Read the model definition and answer for the solid it produces. Units are mm, in the model's axes. A direction names the side the tool comes from. Give positions to 0.01 mm unless a question says otherwise; leave off trailing zeros. Order: outer loops, then holes, each group sorted by start corner. A loop starts at its lowest first (then second) coordinate and runs counter-clockwise, first axis right, second up. Notation, with made-up numbers: M 75.5,59 L 129.5,59 A28 cw 129.5,95 Z; hole C -10.75,-19 d6. An arc over 180 degrees is marked long. Write item = value, one per line. Start each with the question number.
from build123d import *

# Parameters (mm, degrees)
SKETCH_1_W                = 70
SKETCH_1_H                = 30
SKETCH_1_W_2              = 40.6
SKETCH_1_H_2              = 20
EXTRUDE_1_DEPTH           = 51.5
SKETCH_2_R                = 2.1
CUT_EXTRUDE_1_DEPTH       = 52.5
SKETCH_3_R                = 1.6
EXTRUDE_2_DEPTH           = 51.5
SKETCH_17_W               = 155.974555081
SKETCH_17_H               = 17
SKETCH_17_H_2             = 26.5
CUT_EXTRUDE_8_DEPTH       = 31
CUT_EXTRUDE_9_DEPTH       = 52.5
SKETCH_20_W               = 8
SKETCH_20_H               = 10.5
SKETCH_20_H_2             = 2
CUT_EXTRUDE_10_DEPTH      = 208.974555081
CUT_EXTRUDE_10_DEPTH_BACK = 53.025444919
CUT_EXTRUDE_11_DEPTH      = 31


with BuildPart() as part:
    # 草图1 → 凸台-拉伸1 (new body)
    with BuildSketch(Plane(origin=(0, 0, 0), x_dir=(1, 0, 0), z_dir=(0, 1, 0))):
        with Locations((-7.06, 0.32447662)):
            Rectangle(SKETCH_1_W, SKETCH_1_H)
        with Locations((-7.06, 0.32447662)):
            Rectangle(SKETCH_1_W_2, SKETCH_1_H_2, mode=Mode.SUBTRACT)
    extrude(amount=EXTRUDE_1_DEPTH)

    # 草图2 → 切除-拉伸1 (cut, through all)
    with BuildSketch(Plane(origin=(0, 51.5, 0), x_dir=(1, 0, 0), z_dir=(0, 1, 0))):
        with Locations((-31.81, 5.32447662)):
            Circle(SKETCH_2_R)
        with Locations((-31.81, -4.67552338)):
            Circle(SKETCH_2_R)
        with Locations((17.69, -4.67552338)):
            Circle(SKETCH_2_R)
        with Locations((17.69, 5.32447662)):
            Circle(SKETCH_2_R)
    extrude(amount=-CUT_EXTRUDE_1_DEPTH, mode=Mode.SUBTRACT)

    # 草图3 → 凸台-拉伸2 (add)
    with BuildSketch(Plane(origin=(0, 51.5, 0), x_dir=(1, 0, 0), z_dir=(0, 1, 0))):
        with BuildLine():
            Line((-137.06, 10.32447662), (-72.06, 10.32447662))
            Line((-72.06, 10.32447662), (-42.06, 15.32447662))
            Line((-42.06, 15.32447662), (-42.06, -14.67552338))
            Line((-42.06, -14.67552338), (-72.06, -9.67552338))
            Line((-72.06, -9.67552338), (-137.06, -9.67552338))
            ThreePointArc((-137.06, -9.67552338), (-147.06, 0.32447662), (-137.06, 10.32447662))
        make_face()
        with Locations((-137.06, 0.32447662)):
            Circle(SKETCH_3_R, mode=Mode.SUBTRACT)
        with BuildLine():
            Line((57.94, 10.32447662), (102.94, 10.32447662))
            ThreePointArc((102.94, 10.32447662), (112.94, 0.32447662), (102.94, -9.67552338))
            Line((102.94, -9.67552338), (57.94, -9.67552338))
            Line((57.94, -9.67552338), (27.94, -14.67552338))
            Line((27.94, -14.67552338), (27.94, 15.32447662))
            Line((27.94, 15.32447662), (57.94, 10.32447662))
        make_face()
        with Locations((102.94, 0.32447662)):
            Circle(SKETCH_3_R, mode=Mode.SUBTRACT)
    extrude(amount=-EXTRUDE_2_DEPTH)

    # 草图17 → 切除-拉伸8 (cut, through all)
    with BuildSketch(Plane.XY.offset(14.67552338)):
        Polygon((112.94, 45.5), (67.94, 45.5), (67.94, 4), (112.94, 4), (117.101410497, 4), (117.101410497, 45.5), align=None)
        Polygon((-147.034555081, 45.5), (-117.034555081, 45.5), (-102.06, 45.5), (-102.06, 25.5), (-102.06, 4), (-117.034555081, 4), (-147.06, 4), (-149.583075769, 4), (-149.583075769, 45.5), align=None)
        with Locations((-17.047277541, 43)):
            Rectangle(SKETCH_17_W, SKETCH_17_H)
        with Locations((-17.047277541, 13.25)):
            Rectangle(SKETCH_17_W, SKETCH_17_H_2)
    extrude(amount=-CUT_EXTRUDE_8_DEPTH, mode=Mode.SUBTRACT)

    # 草图18 → 切除-拉伸9 (cut, through all)
    with BuildSketch(Plane.XZ):
        Polygon((70.94, -6.21374951), (70.94, -0.06239935), (71.016765061, 6.088471801), (96.014818298, 5.776487199), (95.94, -0.218397725), (95.94, -6.21374951), align=None)
        Polygon((-64.034555081, 4.990640098), (-88.034555081, 4.990640098), (-88.034555081, -5.009335567), (-64.034555081, -5.009335567), (-40.36, -11.056105877), (-40.36, 10.943840585), align=None)
        Polygon((54.94, -0.009359902), (54.94, 4.990640098), (24.94, 10.943840585), (24.94, -0.056159415), (24.974319559, -11.056105877), (54.9555998, -5.009335567), align=None)
        Polygon((-106.034555081, 6.088471801), (-106.034555081, -0.260477592), (-106.014746613, -6.609396085), (-129.01463467, -6.681155163), (-129.034555081, -0.296357219), (-129.034555081, 6.088471801), align=None)
    extrude(amount=-CUT_EXTRUDE_9_DEPTH, mode=Mode.SUBTRACT)

    # 草图20 → 切除-拉伸10 (cut, two sides)
    with BuildSketch(Plane(origin=(-95.034555081, 0, 0), x_dir=(0, 0, -1), z_dir=(1, 0, 0))) as cut_extrude_10_sk:
        with Locations((0.32447662, 15.25)):
            Rectangle(SKETCH_20_W, SKETCH_20_H)
        with Locations((0.32447662, 41.5)):
            Rectangle(SKETCH_20_W, SKETCH_20_H_2)
    extrude(amount=CUT_EXTRUDE_10_DEPTH, mode=Mode.SUBTRACT)
    extrude(cut_extrude_10_sk.sketch, amount=-CUT_EXTRUDE_10_DEPTH_BACK, mode=Mode.SUBTRACT)

    # 草图21 → 切除-拉伸11 (cut, through all)
    with BuildSketch(Plane(origin=(0, 0, -15.32447662), x_dir=(-1, 0, 0), z_dir=(0, 0, -1))):
        Polygon((-55.803056083, 32.5), (94.924677091, 32.5), (95.034555081, 32.5), (95.034555081, 34.5), (88.034555081, 34.5), (-60.94, 34.5), (-60.94, 27.3), align=None)
    extrude(amount=-CUT_EXTRUDE_11_DEPTH, mode=Mode.SUBTRACT)


solid = part.part
1) Find section A-A on y = 6.5. Determine the outline of the cut face in (x, z), plus the area to 3 significant figures.
2) For a pull along Y with two mould halves and no side action, classify faces 1 (the face through (-121, 51.5, -7)), 2 (the face through (-129.2, 45.5, -0.2)), 3 (the face through (-100, 30, 9.676)), 4 (the face through (-18, 26.5, 10)) as pulls with the +Y half, pulls with the -Y half, needs draft (parallel to the pull), parting line crosses it, or undercut.
3) Each of these flat-tipped pins is pushed along its axis until it touches: P1, Ø6.5, axis at y = 48, z = -4.5, coming from the -X side; P2, Ø7.5, axis at x = 65, y = 16.5, coming from the -Z side; P3, Ø4, axis at y = 40.5, z = 9, coming from the +X side; P4, Ø2, axis at x = -80, z = 11, coming from the +Y side. Where does it stop, or does it pass through?
4) Find section C-C on y = 48. Determine the outline of the cut face in (x, z), plus the area to 3 significant figures.
5) Find section B-B on x = -6.5. Determine the outline of the cut face in (y, z), plus the area to 3 significant figures.
6) For faces 5 (the face through (-52.36, 29.46, -7.99)), 6 (the face through (-98, 15, -4.324)), 7 (the face through (-95.035, 13, 4)), determine the directions among +Z, -Z, +X, -X, +Y, -Y from which every point of the face is accessible in a straight line to the end or side of a thin tool.
7) Find the intervals of material crossed by probe 1 along X at (y, z) = (43.5, -8); probe 2 along Y at (x, z) = (101.5, 9); probe 3 along Z at (x, y) = (-137.06, 49.4), in increasing order. Write a range as [from, to].
Numbers:
q1.outline = M -102.06,-10.32 L -95.03,-10.32 L -95.03,9.68 L -102.06,9.68 Z; M 60.94,-10.32 L 67.94,-10.32 L 67.94,9.68 L 60.94,9.68 Z
q1.area = 281 mm2
q2.face_1 = pulls with the +Y half
q2.face_2 = undercut
q2.face_3 = needs draft
q2.face_4 = pulls with the -Y half
q3.P1 = -147.02
q3.P2 = -10.32
q3.P3 = 67.94
q3.P4 = through
q4.outline = M -137.06,-10.32 L -95.03,-10.32 L -95.03,9.68 L -137.06,9.68 A10 ccw Z; M 60.94,-10.32 L 102.94,-10.32 A10 ccw 102.94,9.68 L 60.94,9.68 Z; hole C -137.06,-0.32 d3.2; hole M -129.03,-0.3 L -129.01,-6.68 L -106.01,-6.61 L -106.03,-0.26 L -106.03,6.09 L -129.03,6.09 Z; hole M 70.94,-6.21 L 95.94,-6.21 L 95.94,-0.22 L 96.01,5.78 L 71.02,6.09 L 70.94,-0.06 Z; hole C 102.94,-0.32 d3.2
q4.area = 1,380 mm2
q5.outline = M 26.5,-15.32 L 32.5,-15.32 L 32.5,-10.32 L 26.5,-10.32 Z; M 26.5,9.68 L 32.5,9.68 L 32.5,14.68 L 26.5,14.68 Z
q5.area = 60.0 mm2
q6.face_5 = +Y, -Y
q6.face_6 = +X, -X
q6.face_7 = +Z, -Z, -Y
q7.probe_1 = [-102.06, -95.03], [60.94, 67.94]
q7.probe_2 = [0, 4], [45.5, 51.5]
q7.probe_3 = [-10.32, -1.92], [1.28, 9.68]
